```python
from build123d import *

# Parameters (mm, degrees)
SKETCH2_W               = 4
SKETCH2_H               = 3
SKETCH2_R               = 1.55
SKETCH2_R_2             = 1.6
BOSS_EXTRUDE1_DEPTH     = 8
SKETCH3_W               = 8.237002406
SKETCH3_H               = 20.610649192
CUT_EXTRUDE1_DEPTH      = 43.579337712
CHAMFER1_SIZE           = 3
FILLET4_R               = 1
FILLET5_R               = 0.4
FILLET6_R               = 2
CUT_EXTRUDE2_DEPTH      = 43.579337712
SKETCH7_R               = 2.5
SKETCH7_R_2             = 1.6
BOSS_EXTRUDE2_DEPTH     = 0.5
CHAMFER2_SIZE           = 0.5
CUT_EXTRUDE4_DEPTH      = 43.579337712
CUT_EXTRUDE4_DEPTH_BACK = 43.579337712
SKETCH8_R               = 1.1
FILLET7_R               = 0.6
CHAMFER3_SIZE           = 0.3
CUT_EXTRUDE5_DEPTH      = 1.2
CUT_EXTRUDE5_DEPTH_BACK = 2
CUT_EXTRUDE6_DEPTH      = 10
CUT_EXTRUDE6_DEPTH_BACK = 2
SKETCH11_R              = 1.95


# Some blends are built 0.0001 mm under size
with BuildPart() as part:
    # Sketch1 → Revolve1 (revolve)
    with BuildSketch(Plane.XY, mode=Mode.PRIVATE) as revolve1_sk:
        Polygon((-3.35, 34), (-3.35, 32), (-2.55, 32), (-2.55, 30), (-3.3, 30), (-3.3, 28), (-6.35, 28), (-6.35, 34), align=None)
    revolve(revolve1_sk.sketch.rotate(Axis((0, 0, 0), (0, 1, 0)), 270), axis=Axis((0, 0, 0), (0, 1, 0)))

    # Sketch2 → Boss-Extrude1 (add)
    # profile 1 of 6: a face of its own
    with BuildSketch(Plane(origin=(0, 34, 0), x_dir=(1, 0, 0), z_dir=(0, 1, 0))):
        with Locations((-22, 7.5)):
            Rectangle(SKETCH2_W, SKETCH2_H)
    # profile 2 of 6: a face of its own
    with BuildSketch(Plane(origin=(0, 34, 0), x_dir=(1, 0, 0), z_dir=(0, 1, 0))):
        with Locations((-22, -7.5)):
            Rectangle(SKETCH2_W, SKETCH2_H)
    # profile 3 of 6: a face of its own
    with BuildSketch(Plane(origin=(0, 34, 0), x_dir=(1, 0, 0), z_dir=(0, 1, 0))):
        Polygon((-12, 9), (-20, 9), (-20, 6), (-20, -6), (-20, -9), (-12, -9), (-6.933333333, -5.2), (-8.990544831, -5.2), (-8.990544831, 5.2), (-6.933333333, 5.2), align=None)
        with Locations(Location((-17, -5.5, 0), (0, 0, 270))):
            Circle(SKETCH2_R, mode=Mode.SUBTRACT)
        with Locations(Location((-17, 0, 0), (0, 0, 270))):
            Circle(SKETCH2_R_2, mode=Mode.SUBTRACT)
        with Locations(Location((-17, 5.5, 0), (0, 0, 270))):
            Circle(SKETCH2_R, mode=Mode.SUBTRACT)
    # profile 4 of 6: a face of its own
    with BuildSketch(Plane(origin=(0, 34, 0), x_dir=(1, 0, 0), z_dir=(0, 1, 0))):
        with BuildLine():
            Line((-5.08, 3.81), (-6.933333333, 5.2))
            Line((-6.933333333, 5.2), (-8.990544831, 5.2))
            Line((-8.990544831, 5.2), (-8.990544831, -5.2))
            Line((-8.990544831, -5.2), (-6.933333333, -5.2))
            Line((-6.933333333, -5.2), (-5.08, -3.81))
            ThreePointArc((-5.08, -3.81), (-6.35, 0), (-5.08, 3.81))
        make_face()
    # profile 5 of 6: a face of its own
    with BuildSketch(Plane(origin=(0, 34, 0), x_dir=(1, 0, 0), z_dir=(0, 1, 0))):
        with BuildLine():
            Line((-3.644516429, 5.2), (-6.933333333, 5.2))
            Line((-6.933333333, 5.2), (-5.08, 3.81))
            ThreePointArc((-5.08, 3.81), (-4.417275374, 4.561817431), (-3.644516429, 5.2))
        make_face()
    # profile 6 of 6: a face of its own
    with BuildSketch(Plane(origin=(0, 34, 0), x_dir=(1, 0, 0), z_dir=(0, 1, 0))):
        with BuildLine():
            ThreePointArc((-3.644516429, -5.2), (-4.417275374, -4.561817431), (-5.08, -3.81))
            Line((-5.08, -3.81), (-6.933333333, -5.2))
            Line((-6.933333333, -5.2), (-3.644516429, -5.2))
        make_face()
    extrude(amount=-BOSS_EXTRUDE1_DEPTH)

    # Sketch3 → Cut-Extrude1 (cut, through all)
    with BuildSketch(Plane(origin=(0, 0, 0), x_dir=(1, 0, 0), z_dir=(0, 1, 0))):
        with Locations((5.968501203, -0.12700224)):
            Rectangle(SKETCH3_W, SKETCH3_H)
    extrude(amount=CUT_EXTRUDE1_DEPTH, mode=Mode.SUBTRACT)

    # Chamfer1
    # the kernel refuses this chamfer: 3 mm, written as the material it adds along each edge
    # the kernel refuses this chamfer: 3 mm, written as the material it takes off along each edge
    with BuildSketch(Plane(origin=(0, 26, 0), x_dir=(0.568258769278242, 0, -0.8228499080259886), z_dir=(0.8228499080259886, 0, 0.568258769278242))) as chamfer1_2_piece_1_section:
        Polygon((6.35 + CHAMFER1_SIZE, 0), (6.35, CHAMFER1_SIZE), (6.35, 0), align=None)
    chamfer1_2_piece_1 = revolve(axis=Axis((0, 26, 0), (0, 1, 0)), revolution_arc=249.257786961, mode=Mode.PRIVATE)
    chamfer1_2_piece_1 = split(chamfer1_2_piece_1, bisect_by=Plane(origin=(-8.355666821, 28, 0), z_dir=(0, -1, 0)), keep=Keep.TOP, mode=Mode.PRIVATE)
    add(chamfer1_2_piece_1, mode=Mode.SUBTRACT)

    # Fillet4
    fillet4_edges = [part.edges().sort_by_distance(p)[0] for p in [
        (1.85, 31, 1.754992877),
        (1.85, 31, -1.754992877),
    ]]
    fillet(fillet4_edges, radius=FILLET4_R)

    # Fillet5
    # the kernel refuses this fillet: 0.4 mm, written as the material it takes off along each edge
    with BuildSketch(Plane(origin=(1.684476075, 35.466182436, -2.895693415), x_dir=(-0.8951889914868396, 0, -0.4456867392247326), z_dir=(0, -1, 0))) as fillet5_piece_1:
        with BuildLine():
            CenterArc((0.460657077, 0.399157196), FILLET5_R, 153.532715484, 112.747248008)
            Line((0.10258148, 0.577431892), (0.06677392, 0.595259361))
            ThreePointArc((0.06677392, 0.595259361), (0.061610325, 0.584887966), (-0.039704275, -0.00485495))
            Line((-0.039704275, -0.00485495), (0.002595251, -0.03991572))
            ThreePointArc((0.002595251, -0.03991572), (0.217352283, -0.032941517), (0.432109314, -0.03991572))
            Line((0.432109314, -0.03991572), (0.434704565, 0))
        make_face()
    extrude(amount=3.466182436, mode=Mode.SUBTRACT)
    with BuildSketch(Plane(origin=(1.655788422, 26.609524103, -2.85453406), x_dir=(0.3447573093533237, 0, -0.938691854469536), z_dir=(0, 1, 0))) as fillet5_piece_2:
        with BuildLine():
            CenterArc((0.444952287, 0.384221409), FILLET5_R, 177.1195622, 109.026989702)
            ThreePointArc((0.045457658, 0.404322189), (0.028966063, 0.201459847), (0, 0))
            ThreePointArc((0, 0), (0.278095179, -0.039446477), (0.556190359, 0))
        make_face()
    extrude(amount=3.390475897, mode=Mode.SUBTRACT)
    with BuildSketch(Plane(origin=(1.655788422, 26.609524103, 2.85453406), x_dir=(0.3447573093533235, 0, 0.9386918544695363), z_dir=(0, 1, 0))) as fillet5_piece_3:
        with BuildLine():
            CenterArc((0.444952287, -0.384221409), FILLET5_R, 73.853448098, 109.026989702)
            ThreePointArc((0.045457658, -0.404322189), (0.028966063, -0.201459847), (0, 0))
            ThreePointArc((0, 0), (0.278095179, 0.039446477), (0.556190359, 0))
        make_face()
    extrude(amount=3.390475897, mode=Mode.SUBTRACT)
    with BuildSketch(Plane(origin=(1.684476075, 35.466182436, 2.895693415), x_dir=(-0.8951889914868395, 0, 0.44568673922473334), z_dir=(0, -1, 0))) as fillet5_piece_4:
        with BuildLine():
            CenterArc((0.460657077, -0.399157196), FILLET5_R, 93.720036508, 112.747248008)
            Line((0.10258148, -0.577431892), (0.06677392, -0.595259361))
            ThreePointArc((0.06677392, -0.595259361), (0.061610325, -0.584887966), (-0.039704275, 0.00485495))
            Line((-0.039704275, 0.00485495), (0.002595251, 0.03991572))
            ThreePointArc((0.002595251, 0.03991572), (0.217352283, 0.032941517), (0.432109314, 0.03991572))
            Line((0.432109314, 0.03991572), (0.434704565, 0))
        make_face()
    extrude(amount=3.466182436, mode=Mode.SUBTRACT)

    # Fillet6
    fillet6_edges = [part.edges().sort_by_distance(p)[0] for p in [
        (-20, 30, 6),
        (-20, 30, -6),
    ]]
    fillet(fillet6_edges, radius=FILLET6_R)

    # Sketch5 → Cut-Extrude2 (cut, through all)
    with BuildSketch(Plane(origin=(0, 0, 0), x_dir=(1, 0, 0), z_dir=(0, 1, 0))):
        with BuildLine():
            Line((0, -0.6), (-11, -0.6))
            ThreePointArc((-11, -0.6), (-11.6, 0), (-11, 0.6))
            Line((-11, 0.6), (0, 0.6))
            ThreePointArc((0, 0.6), (0.6, 0), (0, -0.6))
        make_face()
    extrude(amount=CUT_EXTRUDE2_DEPTH, mode=Mode.SUBTRACT)

    # Sketch7 → Boss-Extrude2 (add)
    with BuildSketch(Plane.XZ.offset(-26)):
        with Locations(Location((-17, 0, 0), (0, 0, 90))):
            Circle(SKETCH7_R)
        with Locations(Location((-17, 0, 0), (0, 0, 90))):
            Circle(SKETCH7_R_2, mode=Mode.SUBTRACT)
    extrude(amount=BOSS_EXTRUDE2_DEPTH)

    # Chamfer2
    chamfer2_edges = [part.edges().sort_by_distance(p)[0] for p in [
        (-17, 26, -2.5),
    ]]
    chamfer(chamfer2_edges, length=CHAMFER2_SIZE - 0.0001)  # a hair under: the kernel refuses the full size

    # Sketch8 → Cut-Extrude4 (cut, two sides: drawn at the far end of the back side and taken through both)
    with BuildSketch(Plane.XY.offset(-CUT_EXTRUDE4_DEPTH_BACK)):
        with Locations(Location((-4.5, 31, 0), (0, 0, 321.051593768))):
            Circle(SKETCH8_R)
    extrude(amount=CUT_EXTRUDE4_DEPTH + CUT_EXTRUDE4_DEPTH_BACK, mode=Mode.SUBTRACT)

    # Fillet7
    fillet7_edges = [part.edges().sort_by_distance(p)[0] for p in [
        (-3.644516429, 32.845741182, 5.2),
        (-3.644516429, 32.845741182, -5.2),
        (1.85, 31, 6.074537019),
        (1.85, 31, -6.074537019),
        (-6.933333333, 30.341666667, 5.2),
        (-6.933333333, 30.341666667, -5.2),
    ]]
    fillet(fillet7_edges, radius=FILLET7_R)

    # Chamfer3
    chamfer3_edges = [part.edges().sort_by_distance(p)[0] for p in [
        (-5.355483571, 31.691482364, 0.6),
        (-5.355483571, 31.691482364, -0.6),
    ]]
    chamfer(chamfer3_edges, length=CHAMFER3_SIZE)

    # Sketch10 → Cut-Extrude5 (cut, two sides: drawn at the far end of the back side and taken through both)
    with BuildSketch(Plane.XY.offset(5.2).offset(-CUT_EXTRUDE5_DEPTH_BACK)):
        Polygon((-4.5, 28.575128869), (-2.4, 29.787564435), (-2.4, 32.212435565), (-4.5, 33.424871131), (-6.6, 32.212435565), (-6.6, 29.787564435), align=None)
    extrude(amount=CUT_EXTRUDE5_DEPTH + CUT_EXTRUDE5_DEPTH_BACK, mode=Mode.SUBTRACT)

    # Sketch11 → Cut-Extrude6 (cut, two sides: drawn at the far end of the back side and taken through both)
    with BuildSketch(Plane(origin=(0, 0, -5.2), x_dir=(-1, 0, 0), z_dir=(0, 0, -1)).offset(-CUT_EXTRUDE6_DEPTH_BACK)):
        with Locations(Location((4.5, 31, 0), (0, 0, 120.900188268))):
            Circle(SKETCH11_R)
    extrude(amount=CUT_EXTRUDE6_DEPTH + CUT_EXTRUDE6_DEPTH_BACK, mode=Mode.SUBTRACT)


solid = part.part
```
CAD build for the part. Positions are in the model's coordinates, mm. A direction names the side the tool comes from. Round coordinates to 2 decimals unless told otherwise and drop trailing zeros. Order: outer loops, then holes, each group sorted by start corner. A loop starts at its lowest first (then second) coordinate and runs counter-clockwise, first axis right, second up.
Q1. Two-plate mould, pull along Z, no slides. Class faces 1 (the flat face through (-9.6, 30.1, 7.2)), 2 (the cylindrical face through (-3.93, 31.94, -2.07)), 3 (the flat face through (-23, 30, -6)): pulls with the +Z half, pulls with the -Z half, needs draft (parallel to the pull), parting line crosses it, or undercut.
Q2. Slice it at A-A (y = 31.5). State how many separate pieces and enclosed holes the cut face has, and give its area (3 significant figures).
Q3. Wall check: L1, parallel to Z at x = -6.5, y = 32.75; L2, parallel to Z at x = -16, y = 32.25; L3, parallel to Y at x = -4.5, z = -2.15. Give the ranges that are in metal, low to high.
Q4. Drop flat-ended pins along their axis: pin 1 (1.5 mm diameter, centred on x = -5.5, y = 30.5, fed in from +Z); pin 2 (2 mm diameter, centred on x = -4, y = 31.5, fed in from -Z); pin 3 (5 mm diameter, centred on x = -4.5, y = 31, fed in from -Z). Give the stop position or say it passes through.
Q5. Which spindle directions (+Z, -Z, +X, -X, +Y, -Y) get a long thin tool onto all of the face, cutting with end or side? Do faces 4 (the flat face through (-6.6, 31, 4)), 5 (the cylindrical face through (-20.6, 29.94, -5.43)), 6 (the flat face through (-8, 31, -0.6)). Say none if no direction does.
Q6. Slice it at B-B (z = -7.5). Write the cut outline in (x, y), and give its area (3 significant figures).
Results below:
1. face 1: pulls with the +Z half
1. face 2: needs draft
1. face 3: undercut
2. separate pieces: 3
2. enclosed holes: 3
2. area: 262 mm2
3. L1: z = -5.2 to -0.6, 0.6 to 5.2
3. L2: z = -9 to -6.68, -4.32 to -1.25, 1.25 to 4.32, 6.68 to 9
3. L3: y = 28 to 29.9, 32.1 to 34
4. pin 1: stops at z = 3.2
4. pin 2: stops at z = -3.2
4. pin 3: stops at z = -6.03
5. face 4: +Z
5. face 5: -X, +Y, -Y
5. face 6: +X, +Y, -Y
6. outline: (-24, 26) - (-10, 26) - (-10, 34) - (-24, 34) - close
6. area: 112 mm2
